from build123d import *

# Parameters (mm, degrees)
SKETCH1_W               = 25.4
SKETCH1_H               = 12.7
BOSS_EXTRUDE1_DEPTH     = 127
SKETCH4_W               = 22.86
SKETCH4_H               = 10.16
CUT_EXTRUDE1_DEPTH      = 128
SKETCH5_R               = 1.8034
CUT_EXTRUDE2_DEPTH      = 1
CUT_EXTRUDE2_DEPTH_BACK = 13.7
SKETCH6_R               = 1.524
CUT_EXTRUDE3_DEPTH      = 1
CUT_EXTRUDE3_DEPTH_BACK = 13.7
SKETCH7_W               = 25.4
SKETCH7_H               = 12.7
SKETCH7_W_2             = 22.86
SKETCH7_H_2             = 10.16
BOSS_EXTRUDE2_DEPTH     = 25.4
CUT_EXTRUDE4_REACH      = 154.4
SKETCH8_W               = 1.27
SKETCH8_H               = 10.16
BOSS_EXTRUDE3_START     = -50.8
SKETCH9_W               = 24.13
SKETCH9_H               = 10.16
BOSS_EXTRUDE3_DEPTH     = 76.2


with BuildPart() as part:
    # Sketch1 → Boss-Extrude1 (new body)
    with BuildSketch(Plane.XY):
        Rectangle(SKETCH1_W, SKETCH1_H)
    extrude(amount=BOSS_EXTRUDE1_DEPTH)

    # Sketch4 → Cut-Extrude1 (cut, through all)
    with BuildSketch(Plane(origin=(0, 0, 0), x_dir=(-1, 0, 0), z_dir=(0, 0, -1))):
        Rectangle(SKETCH4_W, SKETCH4_H)
    extrude(amount=-CUT_EXTRUDE1_DEPTH, mode=Mode.SUBTRACT)

    # Sketch5 → Cut-Extrude2 (cut, two sides)
    with BuildSketch(Plane(origin=(0, 6.35, 0), x_dir=(1, 0, 0), z_dir=(0, 1, 0))) as cut_extrude2_sk:
        with Locations((-5.588, -123.698)):
            Circle(SKETCH5_R)
        with Locations((5.5372, -123.698)):
            Circle(SKETCH5_R)
    extrude(amount=CUT_EXTRUDE2_DEPTH, mode=Mode.SUBTRACT)
    extrude(cut_extrude2_sk.sketch, amount=-CUT_EXTRUDE2_DEPTH_BACK, mode=Mode.SUBTRACT)

    # Sketch6 → Cut-Extrude3 (cut, two sides)
    with BuildSketch(Plane(origin=(0, -6.35, 0), x_dir=(-1, 0, 0), z_dir=(0, -1, 0))) as cut_extrude3_sk:
        with Locations((4.445, -6.35)):
            Circle(SKETCH6_R)
        with Locations((-4.4704, -6.35)):
            Circle(SKETCH6_R)
        with Locations((0, -1.905)):
            Circle(SKETCH6_R)
        with Locations((0, -10.795)):
            Circle(SKETCH6_R)
    extrude(amount=CUT_EXTRUDE3_DEPTH, mode=Mode.SUBTRACT)
    extrude(cut_extrude3_sk.sketch, amount=-CUT_EXTRUDE3_DEPTH_BACK, mode=Mode.SUBTRACT)

    # Sketch7 → Boss-Extrude2 (add)
    with BuildSketch(Plane(origin=(0, 0, 0), x_dir=(-1, 0, 0), z_dir=(0, 0, -1))):
        Rectangle(SKETCH7_W, SKETCH7_H)
        Rectangle(SKETCH7_W_2, SKETCH7_H_2, mode=Mode.SUBTRACT)
    extrude(amount=BOSS_EXTRUDE2_DEPTH)

    # Sketch8 → Cut-Extrude4 (cut, up to next)
    with BuildSketch(Plane(origin=(0, 0, -25.4), x_dir=(-1, 0, 0), z_dir=(0, 0, -1)), mode=Mode.PRIVATE) as cut_extrude4_sk1:
        with Locations((-12.065, 0)):
            Rectangle(SKETCH8_W, SKETCH8_H)
    cut_extrude4_tool1 = extrude(cut_extrude4_sk1.sketch, amount=-CUT_EXTRUDE4_REACH, mode=Mode.PRIVATE) & part.part
    add(cut_extrude4_tool1.solids().sort_by_distance((12.065, 0, -25.4))[0], mode=Mode.SUBTRACT)

    # Sketch9 → Boss-Extrude3 (add)
    with BuildSketch(Plane(origin=(0, 0, -25.4), x_dir=(-1, 0, 0), z_dir=(0, 0, -1)).offset(BOSS_EXTRUDE3_START)):
        with Locations((-0.635, 0)):
            Rectangle(SKETCH9_W, SKETCH9_H)
    extrude(amount=-BOSS_EXTRUDE3_DEPTH)


solid = part.part
Input: part model. Units: mm. Frame: model coordinates. A direction names the side the tool comes from. Round coordinates to 2 decimals unless told otherwise and drop trailing zeros. Order: outer loops, then holes, each group sorted by start corner. A loop starts at its lowest first (then second) coordinate and runs counter-clockwise, first axis right, second up. Notation, with made-up numbers: (1.5, 86.25) - (9.5, 86.25) arc R4 ccw to (9.5, 91.25) - close; hole circle Ø7 at (49, -3.75). An arc over 180 degrees is marked (long way). Answer as a JSON object with one key per item and string values. Group by question number.
(1) Cut plane B-B (x = 0.25). Return loops of the section in (y, z).
(2) Draft query along X for faces 1 (the face through (12.7, 0, 52)), 2 (the face through (0, -6.35, 52)), 3 (the face through (-5.82, -5.71, 121.91)). Return one class per face: released by +X, released by -X, zero draft, split by the parting line, or undercut.
(3) Cut plane C-C (y = 3.5). Return loops of the section in (x, z), then the cut area to 3 significant figures.
(4) Cut plane D-D (z = -10.5). Return loops of the section in (x, y), then the cut area to 3 significant figures.
(5) Pin query (flat end, axial travel): P1, Ø1.8, axis at x = -4.445, z = 6.35, coming from the +Y side; P2, Ø3, axis at x = 8.5, y = -2, coming from the +Z side; P3, Ø2, axis at x = -7, y = 3.5, coming from the -Z side; P4, Ø6, axis at y = 1.5, z = -1, coming from the +X side. Return the tip coordinate at first contact, or that it passes through.
(6) Material intervals for probe 1 along Y at (x, z) = (10, 104.5); probe 2 along Z at (x, y) = (-10.75, 1); probe 3 along X at (y, z) = (2.75, 10), sorted ascending. Write a range as from..to.
(7) Reachability of faces 4 (the face through (-11.43, 0, 0)), 5 (the face through (-11.43, 0, 114)), 6 (the face through (-5.82, 5.72, 121.91)) from +Z, -Z, +X, -X, +Y, -Y: full face, straight path, thin tool, end or side. Return the list, or none.
(8) Cut plane A-A (z = 6.35). Return loops of the section in (x, y).
Here are the results:
{
 "1": {"outline": "(-6.35, -25.4) - (-5.08, -25.4) - (-5.08, 0.4) - (-6.35, 0.4) - close; (-6.35, 3.41) - (-5.08, 3.41) - (-5.08, 9.29) - (-6.35, 9.29) - close; (-6.35, 12.3) - (-5.08, 12.3) - (-5.08, 25.4) - (5.08, 25.4) - (5.08, 12.3) - (6.35, 12.3) - (6.35, 127) - (5.08, 127) - (5.08, 101.6) - (-5.08, 101.6) - (-5.08, 127) - (-6.35, 127) - close; (5.08, -25.4) - (6.35, -25.4) - (6.35, 0.4) - (5.08, 0.4) - close; (5.08, 3.41) - (6.35, 3.41) - (6.35, 9.29) - (5.08, 9.29) - close"},
 "2": {"face 1": "released by +X", "face 2": "zero draft", "face 3": "undercut"},
 "3": {"outline": "(-12.7, -25.4) - (-11.43, -25.4) - (-11.43, 25.4) - (12.7, 25.4) - (12.7, 101.6) - (-11.43, 101.6) - (-11.43, 127) - (-12.7, 127) - close", "area": "2,030 mm^2"},
 "4": {"outline": "(-12.7, -6.35) - (12.7, -6.35) - (12.7, -5.08) - (-11.43, -5.08) - (-11.43, 5.08) - (12.7, 5.08) - (12.7, 6.35) - (-12.7, 6.35) - close", "area": "77.4 mm^2"},
 "5": {"P1": "passes through", "P2": "stops at z = 101.6", "P3": "stops at z = 25.4", "P4": "stops at x = -11.43"},
 "6": {"probe 1": "y = -6.35..-5.08, 5.08..6.35", "probe 2": "z = 25.4..101.6", "probe 3": "x = -12.7..-11.43"},
 "7": {"face 4": "-Z, +X", "face 5": "+Z, +X", "face 6": "+Y, -Y"},
 "8": {"outline": "(-12.7, -6.35) - (-5.97, -6.35) - (-5.97, -5.08) - (-11.43, -5.08) - (-11.43, 5.08) - (-5.97, 5.08) - (-5.97, 6.35) - (-12.7, 6.35) - close; (-2.92, -6.35) - (2.95, -6.35) - (2.95, -5.08) - (-2.92, -5.08) - close; (-2.92, 5.08) - (2.95, 5.08) - (2.95, 6.35) - (-2.92, 6.35) - close; (5.99, -6.35) - (12.7, -6.35) - (12.7, -5.08) - (5.99, -5.08) - close; (5.99, 5.08) - (12.7, 5.08) - (12.7, 6.35) - (5.99, 6.35) - close"}
}
